```python
from build123d import *

# Parameters (mm, degrees)
SKETCH1_W           = 16
SKETCH1_H           = 16
BOSS_EXTRUDE1_DEPTH = 2
FILLET1_R           = 1
SKETCH2_R           = 1.75
CUT_EXTRUDE1_DEPTH  = 3


with BuildPart() as part:
    # Sketch1 → Boss-Extrude1 (new body)
    with BuildSketch(Plane(origin=(0, 0, 0), x_dir=(1, 0, 0), z_dir=(0, 1, 0))):
        Rectangle(SKETCH1_W, SKETCH1_H)
    extrude(amount=BOSS_EXTRUDE1_DEPTH)

    # Fillet1
    fillet1_edges = [part.edges().sort_by_distance(p)[0] for p in [
        (8, 1, 8),
        (-8, 1, 8),
        (-8, 1, -8),
        (8, 1, -8),
    ]]
    fillet(fillet1_edges, radius=FILLET1_R)

    # Sketch2 → Cut-Extrude1 (cut, through all)
    with BuildSketch(Plane(origin=(0, 2, 0), x_dir=(1, 0, 0), z_dir=(0, 1, 0))):
        Circle(SKETCH2_R)
    extrude(amount=-CUT_EXTRUDE1_DEPTH, mode=Mode.SUBTRACT)


solid = part.part
```
Can you work these out from the model? Positions are in its coordinate system, mm. Round coordinates to 2 decimals unless told otherwise and drop trailing zeros. Loops run counter-clockwise (first coordinate to the right, second up) from the corner with the lowest first, then second, coordinate; pieces in that order, holes last. Notation, with made-up numbers: M 89.5,26 L 95.5,26 A27 ccw 95.5,50 Z; hole C 77.25,7 d1. An arc over 180 degrees is marked long. Answer in a Markdown table with one row per item.
1. I'm going to push flat-ended pins straight in: pin 1 Ø3 at (x, z) = (0, 0) entering from +Y; pin 2 Ø8 at (x, z) = (-3.5, -3.5) entering from -Y. Where does each tip first touch, or does it pass through?
Established:
| item | result |
|---|---|
| pin 1 | through |
| pin 2 | y = 0 |
2. If we section it at B-B, the plane y = 0.4: Please give me the cut outline in (x, z), plus the area to 3 significant figures.
Established:
| item | result |
|---|---|
| outline | M -8,-7 A1 ccw -7,-8 L 7,-8 A1 ccw 8,-7 L 8,7 A1 ccw 7,8 L -7,8 A1 ccw -8,7 Z; hole C 0,0 d3.5 |
| area | 246 mm² |
3. If we section it at C-C, the plane z = 0: Please give me the cut outline in (x, y).
Established:
| item | result |
|---|---|
| outline | M -8,0 L -1.75,0 L -1.75,2 L -8,2 Z; M 1.75,0 L 8,0 L 8,2 L 1.75,2 Z |
4. Please list where these lines run through material, in increasing order: line 1 (X direction, y = 0.7, z = 0); line 2 (Z direction, x = 0.75, y = 1.4). Write a range as from..to.
Established:
| item | result |
|---|---|
| line 1 | -8..-1.75, 1.75..8 |
| line 2 | -8..-1.58, 1.58..8 |
5. If we section it at A-A, the plane x = 0: Please give me the cut outline in (y, z).
Established:
| item | result |
|---|---|
| outline | M 0,-8 L 2,-8 L 2,-1.75 L 0,-1.75 Z; M 0,1.75 L 2,1.75 L 2,8 L 0,8 Z |
